```python
from build123d import *

# Parameters (mm, degrees)
F1_DEPTH = 3.81
F2_DEPTH = 3.81
F3_DEPTH = 3.81
F4_DEPTH = 3.81
F5_DEPTH = 3.81
F6_DEPTH = 3.81


with BuildPart() as f1:
    # F0 (on Top) → F1 (new body)
    with BuildSketch(Plane.XY):
        Polygon((57.15, -38.1), (57.15, 38.1), (-57.15, 38.1), (-57.15, -38.1), (-31.75, -63.5), (0, -63.5), (31.75, -63.5), align=None)
    extrude(amount=F1_DEPTH)

    # F2 (add): a face of the model
    f2_faces = [f1.faces().sort_by_distance(p)[0] for p in [
        (0, -63.5, 1.905),
    ]]
    extrude(f2_faces, amount=F2_DEPTH)

    # F3 (add): a face of the model
    f3_faces = [f1.faces().sort_by_distance(p)[0] for p in [
        (44.45, -50.8, 1.905),
    ]]
    extrude(f3_faces, amount=F3_DEPTH)

    # F4 (add): a face of the model
    f4_faces = [f1.faces().sort_by_distance(p)[0] for p in [
        (-44.45, -50.8, 1.905),
    ]]
    extrude(f4_faces, amount=F4_DEPTH)

    # F5 (add): a face of the model
    f5_faces = [f1.faces().sort_by_distance(p)[0] for p in [
        (-57.15, 0, 1.905),
    ]]
    extrude(f5_faces, amount=F5_DEPTH)

    # F6 (add): a face of the model
    f6_faces = [f1.faces().sort_by_distance(p)[0] for p in [
        (57.15, 0, 1.905),
    ]]
    extrude(f6_faces, amount=F6_DEPTH)


solid = f1.part
```
Check sheet for the modelled part. Datum: model origin and axes. Units: mm. Coordinates: 2 decimals unless noted, no trailing zeros. Write each loop counter-clockwise with the first axis right and the second up, starting at its lowest first coordinate (ties: lowest second). Pieces come first, ordered by that corner, then holes. Notation, with made-up numbers: (86.5, 35) -> (130.5, 35) arc R11 ccw to (130.5, 49) -> close; hole circle Ø9 at (-21.75, 80.25). An arc over 180 degrees is marked (long way). Use a Markdown table: item, result.
1. Sectioned sample at B-B (x = -51). Enter the section's corners in (y, z).
Reported:
| item | result |
|---|---|
| outline | (-49.64, 0) -> (38.1, 0) -> (38.1, 3.81) -> (-49.64, 3.81) -> close |
2. Sectioned sample at C-C (x = 53.5). Enter the section's corners in (y, z).
Reported:
| item | result |
|---|---|
| outline | (-47.14, 0) -> (38.1, 0) -> (38.1, 3.81) -> (-47.14, 3.81) -> close |
3. Go/stop test with flat-tipped pins: pin 1 Ø1.9 at (x, z) = (-59, 1.5) entering from -Y; pin 2 Ø1.9 at (x, z) = (59.5, 1.5) entering from -Y. Record where each tip stops, or that it passes through.
Reported:
| item | result |
|---|---|
| pin 1 | stops at y = -42.59 |
| pin 2 | stops at y = -42.09 |
4. Scan lines: line 1 along X through (y, z) = (-44, 2.3); line 2 along X through (y, z) = (-56.5, 3.35); line 3 along Y through (x, z) = (50.5, 2.8). Record each from-to range of solid material in increasing order.
Reported:
| item | result |
|---|---|
| line 1 | x = -56.64 to 56.64 |
| line 2 | x = -44.14 to 44.14 |
| line 3 | y = -50.14 to 38.1 |
5. Sectioned sample at A-A (z = 2.2). Enter the section's corners in (x, y).
Reported:
| item | result |
|---|---|
| outline | (-60.96, -38.1) -> (-57.15, -38.1) -> (-59.84, -40.79) -> (-34.44, -66.19) -> (-31.75, -63.5) -> (-31.75, -67.31) -> (31.75, -67.31) -> (31.75, -63.5) -> (34.44, -66.19) -> (59.84, -40.79) -> (57.15, -38.1) -> (60.96, -38.1) -> (60.96, 38.1) -> (-60.96, 38.1) -> close |
6. Release check for a two-part mould opening along Y. For faces 1 (the flat face through (-1, 38.1, 2)), 2 (the flat face through (-1, -15, 3.81)), 3 (the flat face through (-59, -38.1, 2)) record: pulls with the +Y half, pulls with the -Y half, needs draft (parallel to the pull), parting line crosses it, or undercut.
Reported:
| item | result |
|---|---|
| face 1 | pulls with the +Y half |
| face 2 | needs draft |
| face 3 | undercut |
